from build123d import *

# Parameters (mm, degrees)
BOSS_EXTRUDE1_DEPTH     = 5
CUT_EXTRUDE1_DEPTH      = 53.75142939
CUT_EXTRUDE1_DEPTH_BACK = 53.75142939
SKETCH2_R               = 1.75
BOSS_EXTRUDE2_START     = 0.5
SKETCH3_R               = 2.5
SKETCH3_R_2             = 1.75
BOSS_EXTRUDE2_DEPTH     = 0.5
SKETCH5_R               = 3
CUT_EXTRUDE2_DEPTH      = 2


with BuildPart() as part:
    # Sketch1 → Boss-Extrude1 (new body)
    with BuildSketch(Plane.XY):
        with BuildLine():
            Line((23.11684397, 8), (36.88315603, 8))
            Line((36.88315603, 8), (46.90520921, 5.744848006))
            ThreePointArc((46.90520921, 5.744848006), (51.591551748, -2.466147717), (42.989140572, -6.387981358))
            Line((42.989140572, -6.387981358), (34.244441462, -2.658908715))
            ThreePointArc((34.244441462, -2.658908715), (30, -2), (25.755558538, -2.658908715))
            Line((25.755558538, -2.658908715), (17.05409045, -6.415729603))
            ThreePointArc((17.05409045, -6.415729603), (8.36828995, -2.480244081), (13.111532947, 5.792169261))
            Line((13.111532947, 5.792169261), (23.11684397, 8))
        make_face()
    extrude(amount=BOSS_EXTRUDE1_DEPTH)

    # Sketch2 → Cut-Extrude1 (cut, two sides: drawn at the far end of the back side and taken through both)
    with BuildSketch(Plane.XY.offset(5).offset(-CUT_EXTRUDE1_DEPTH_BACK)):
        with Locations((45.5, -0.5)):
            Circle(SKETCH2_R)
        with Locations((14.5, -0.5)):
            Circle(SKETCH2_R)
        with Locations((26, 3)):
            Circle(SKETCH2_R)
        with Locations((34, 3)):
            Circle(SKETCH2_R)
    extrude(amount=CUT_EXTRUDE1_DEPTH + CUT_EXTRUDE1_DEPTH_BACK, mode=Mode.SUBTRACT)

    # Sketch3 → Boss-Extrude2 (add)
    with BuildSketch(Plane.XY.offset(5).offset(BOSS_EXTRUDE2_START)):
        with Locations((14.5, -0.5)):
            Circle(SKETCH3_R)
        with Locations((14.5, -0.5)):
            Circle(SKETCH3_R_2, mode=Mode.SUBTRACT)
    extrude(amount=-BOSS_EXTRUDE2_DEPTH)

    # Sketch5 → Cut-Extrude2 (cut)
    with BuildSketch(Plane.XY.offset(5)):
        with Locations((26, 3)):
            Circle(SKETCH5_R)
        with Locations((34, 3)):
            Circle(SKETCH5_R)
        with Locations((45.5, -0.5)):
            Circle(SKETCH5_R)
    extrude(amount=-CUT_EXTRUDE2_DEPTH, mode=Mode.SUBTRACT)


solid = part.part
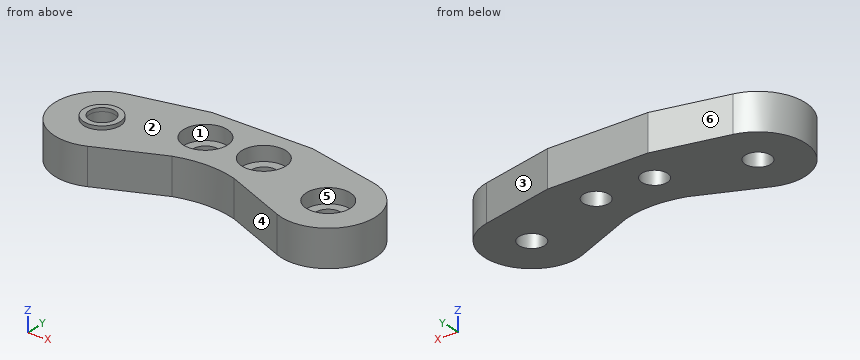
Geometry: final body of the model. Coordinates: model frame, mm. Face numbers are marked on the shaded views. A direction names the side the tool comes from. Coordinates: 2 decimals unless noted, no trailing zeros. Order: outer loops, then holes, each group sorted by start corner. A loop starts at its lowest first (then second) coordinate and runs counter-clockwise, first axis right, second up.
1) Draft query along X for the marked faces 1, 2 and 3. Return one class per face: released by +X, released by -X, zero draft, split by the parting line, or undercut.
Result sheet:
face 1: undercut
face 2: zero draft
face 3: released by +X
2) Section B-B (z = 4.55). Return loops of the section in (x, y), then the cut area to 3 significant figures.
Result sheet:
outline: (13.11, 5.79) arc R6.44 ccw (long way) to (17.05, -6.42) - (25.76, -2.66) arc R14 cw to (34.24, -2.66) - (42.99, -6.39) arc R6.4 ccw (long way) to (46.91, 5.74) - (36.88, 8) - (23.12, 8) - close; hole circle Ø3.5 at (14.5, -0.5); hole circle Ø6 at (26, 3); hole circle Ø6 at (34, 3); hole circle Ø6 at (45.5, -0.5)
area: 399 mm2
3) Section C-C (y = -6). Return loops of the section in (x, z).
Result sheet:
outline: (11.14, 0) - (18.02, 0) - (18.02, 5) - (11.14, 5) - close; (42.08, 0) - (48.77, 0) - (48.77, 5) - (42.08, 5) - close
4) Set-up query: the marked faces 4, 5 and 6. Return all of +Z, -Z, +X, -X, +Y, -Y with unobstructed straight access to the full face (end or side cutting, diameter ignored); none if empty.
Result sheet:
face 4: +Z, -Z, -Y
face 5: +Z
face 6: +Z, -Z, -X, +Y
5) Ray query, probe 1 along X at (y, z) = (-0.5, 1.9); probe 2 along Y at (x, z) = (14.5, 5.1); probe 3 along X at (y, z) = (3.5, 0.7). Return the intervals inside material, ascending.
Result sheet:
probe 1: x = 8.06 to 12.75, 16.25 to 43.75, 47.25 to 51.9
probe 2: y = -3 to -2.25, 1.25 to 2
probe 3: x = 9.45 to 24.32, 27.68 to 32.32, 35.68 to 50.5
6) Section A-A (y = -0.5). Return loops of the section in (x, z).
Result sheet:
outline: (8.06, 0) - (12.75, 0) - (12.75, 5.5) - (12, 5.5) - (12, 5) - (8.06, 5) - close; (16.25, 0) - (43.75, 0) - (43.75, 3) - (42.5, 3) - (42.5, 5) - (17, 5) - (17, 5.5) - (16.25, 5.5) - close; (47.25, 0) - (51.9, 0) - (51.9, 5) - (48.5, 5) - (48.5, 3) - (47.25, 3) - close
7) First-contact query: P1, Ø3, axis at x = 14.5, y = -0.5, coming from the -Z side; P2, Ø4, axis at x = 34, y = 3, coming from the +Z side; P3, Ø5, axis at x = 27, y = 6.5, coming from the -Z side; P4, Ø2, axis at x = 42, z = 1, coming from the -Y side. Flat tips, straight axial feed; report the tip coordinate or a pass-through.
Result sheet:
P1: passes through
P2: stops at z = 3
P3: stops at z = 0
P4: stops at y = -6.39
8) Section D-D (x = 45.5). Return loops of the section in (y, z).
Result sheet:
outline: (-6.9, 0) - (-2.25, 0) - (-2.25, 3) - (-3.5, 3) - (-3.5, 5) - (-6.9, 5) - close; (1.25, 0) - (6.06, 0) - (6.06, 5) - (2.5, 5) - (2.5, 3) - (1.25, 3) - close
